Read the model definition and answer for the solid it produces. Units are mm, in the model's axes. Face numbers are marked on the shaded views. Coordinates: 2 decimals unless noted, no trailing zeros. Write each loop counter-clockwise with the first axis right and the second up, starting at its lowest first coordinate (ties: lowest second). Pieces come first, ordered by that corner, then holes. Notation, with made-up numbers: M 9.5,-10.75 L 49.5,-10.75 A16 cw 49.5,20.25 Z; hole C 74.25,89 d7. An arc over 180 degrees is marked long. Use a Markdown table: item, result. Add a question column.
from build123d import *

# Parameters (mm, degrees)
SKETCH2_R           = 2
BOSS_EXTRUDE1_DEPTH = 10


with BuildPart() as part:
    # Sketch2 → Boss-Extrude1 (new body)
    with BuildSketch(Plane.XY):
        Polygon((0, 2.5), (0.585270966, 2.942355841), (0.956708581, 2.309698831), (1.666710699, 2.494408837), (1.767766953, 1.767766953), (2.494408837, 1.666710699), (2.309698831, 0.956708581), (2.942355841, 0.585270966), (2.5, 0), (2.942355841, -0.585270966), (2.309698831, -0.956708581), (2.494408837, -1.666710699), (1.767766953, -1.767766953), (1.666710699, -2.494408837), (0.956708581, -2.309698831), (0.585270966, -2.942355841), (0, -2.5), (-0.585270966, -2.942355841), (-0.956708581, -2.309698831), (-1.666710699, -2.494408837), (-1.767766953, -1.767766953), (-2.494408837, -1.666710699), (-2.309698831, -0.956708581), (-2.942355841, -0.585270966), (-2.5, 0), (-2.942355841, 0.585270966), (-2.309698831, 0.956708581), (-2.494408837, 1.666710699), (-1.767766953, 1.767766953), (-1.666710699, 2.494408837), (-0.956708581, 2.309698831), (-0.585270966, 2.942355841), align=None)
        Circle(SKETCH2_R, mode=Mode.SUBTRACT)
    extrude(amount=BOSS_EXTRUDE1_DEPTH)


solid = part.part
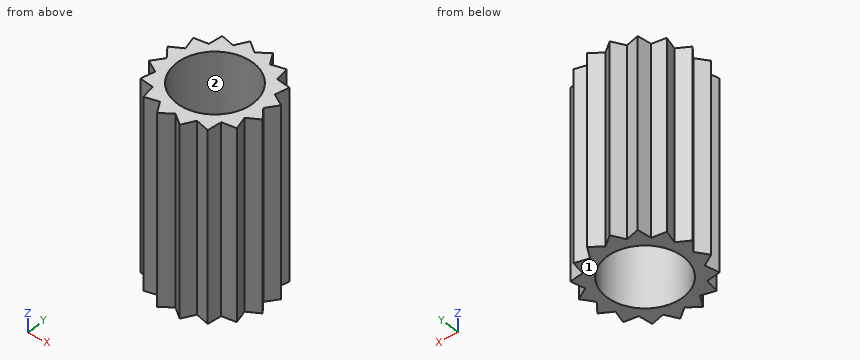
Item 1: Determine the mould class of the marked faces 1 and 2 for opening direction Y: pulls with the +Y half, pulls with the -Y half, needs draft (parallel to the pull), parting line crosses it, or undercut.
Item 2: Find section C-C on x = 0.7. Give the vertices of the cut face in (y, z), then the cut area to 3 significant figures.
Item 3: Consider probe 1 along X at (y, z) = (0.45, 9.25); probe 2 along Y at (x, z) = (0.4, 6). Determine where each line is inside the solid, lowest interval first.
Item 4: Find section B-B on y = 0.75. Give the vertices of the cut face in (x, z), then the cut area to 3 significant figures.
Item 5: Each of these flat-tipped pins is pushed along its axis until it touches: pin 1 (2 mm diameter, centred on x = -0.5, y = -1.5, fed in from -Z); pin 2 (3 mm diameter, centred on x = 0, y = 0, fed in from +Z); pin 3 (2 mm diameter, centred on x = -2.5, z = 4, fed in from -Y). Where does it stop, or does it pass through?
Geometry says:
| question | item | result |
|---|---|---|
| 1 | face 1 | needs draft |
| 1 | face 2 | undercut |
| 2 | outline | M -2.75,0 L -1.87,0 L -1.87,10 L -2.75,10 Z; M 1.87,0 L 2.75,0 L 2.75,10 L 1.87,10 Z |
| 2 | area | 17.5 mm2 |
| 3 | probe 1 | x = -2.84 to -1.95, 1.95 to 2.84 |
| 3 | probe 2 | y = -2.8 to -1.96, 1.96 to 2.8 |
| 4 | outline | M -2.66,0 L -1.85,0 L -1.85,10 L -2.66,10 Z; M 1.85,0 L 2.66,0 L 2.66,10 L 1.85,10 Z |
| 4 | area | 16.2 mm2 |
| 5 | pin 1 | stops at z = 0 |
| 5 | pin 2 | passes through |
| 5 | pin 3 | stops at y = -2.49 |
